from build123d import *

# Parameters (mm, degrees)
EXTRUDE002_DEPTH = 3
SKETCH001_W      = 60
SKETCH001_H      = 3
EXTRUDE001_DEPTH = 20
SKETCH_W         = 60
SKETCH_H         = 23
SKETCH_R         = 2.5
EXTRUDE_DEPTH    = 3


with BuildPart() as extrude002:
    # Face002 → Extrude002 (new body)
    with BuildSketch(Plane(origin=(30, 0, 17.604991), x_dir=(1, 0, 0), z_dir=(0, 1, 0))):
        with BuildLine():
            Line((-1, -5.395009), (1, -5.395009))
            Line((1, -5.395009), (1, 4.604991))
            ThreePointArc((1, 4.604991), (0, 5.604991), (-1, 4.604991))
            Line((-1, 4.604991), (-1, -5.395009))
        make_face()
    extrude(amount=EXTRUDE002_DEPTH)


with BuildPart() as cut:
    # Sketch001 (on Face7 of Extrude) → Extrude001 (new body)
    with BuildSketch(Plane.XY.offset(3)):
        with Locations((30, 1.5)):
            Rectangle(SKETCH001_W, SKETCH001_H)
    extrude(amount=EXTRUDE001_DEPTH)

    # Cut: cut Extrude002
    add(extrude002.part, mode=Mode.SUBTRACT)


with BuildPart() as fusion:
    # Sketch → Extrude (new body)
    with BuildSketch(Plane.XY):
        with Locations((30, 11.5)):
            Rectangle(SKETCH_W, SKETCH_H)
        with Locations((30, 13)):
            Circle(SKETCH_R, mode=Mode.SUBTRACT)
    extrude(amount=EXTRUDE_DEPTH)

    # Fusion: union Cut
    add(cut.part)


solid = fusion.part
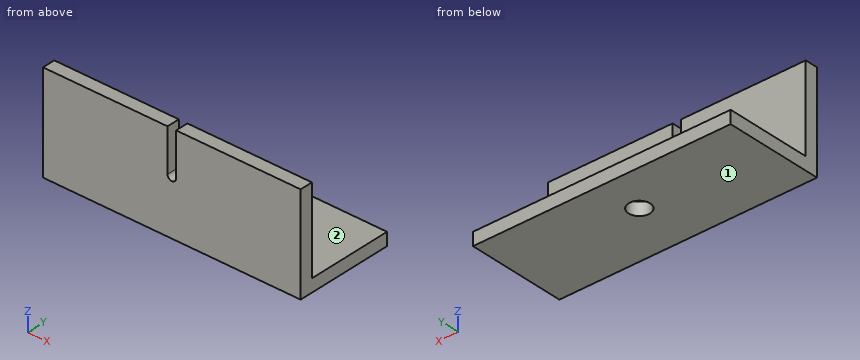
Source: CAD feature listing. Evaluate the final solid. Frame: model axes, mm. Face numbers are marked on the shaded views. A direction names the side the tool comes from. Give positions to 0.01 mm unless a question says otherwise; leave off trailing zeros. Order: outer loops, then holes, each group sorted by start corner. A loop starts at its lowest first (then second) coordinate and runs counter-clockwise, first axis right, second up. Notation, with made-up numbers: (81.5, 21.5) -> (93.5, 21.5) arc R29 cw to (93.5, 52.5) -> close; hole circle Ø9 at (65.5, 68). An arc over 180 degrees is marked (long way). Use a Markdown table: item, result.
1) Contact query for flat-ended pins moving along their axis: P1, Ø8, axis at x = 30, y = 13, coming from the +Z side; P2, Ø10, axis at x = 14.5, z = 11.5, coming from the +Y side; P3, Ø2.5, axis at y = 2, z = 20, coming from the -X side. Output: stop coordinate, or through.
Answer list:
| item | result |
|---|---|
| P1 | z = 3 |
| P2 | y = 3 |
| P3 | x = 0 |
2) Reachability of the marked faces 1 and 2 from +Z, -Z, +X, -X, +Y, -Y: full face, straight path, thin tool, end or side. Return the list, or none.
Answer list:
| item | result |
|---|---|
| face 1 | -Z, +X, -X, +Y, -Y |
| face 2 | +Z, +X, -X, +Y |
3) Section query B-B, the plane x = 30. Return the cut outline in (y, z), then the cut area to 3 significant figures.
Answer list:
| item | result |
|---|---|
| outline | (0, 0) -> (10.5, 0) -> (10.5, 3) -> (3, 3) -> (3, 12) -> (0, 12) -> close; (15.5, 0) -> (23, 0) -> (23, 3) -> (15.5, 3) -> close |
| area | 81.0 mm² |
4) Section query C-C, the plane y = 13. Return the cut outline in (x, z).
Answer list:
| item | result |
|---|---|
| outline | (0, 0) -> (27.5, 0) -> (27.5, 3) -> (0, 3) -> close; (32.5, 0) -> (60, 0) -> (60, 3) -> (32.5, 3) -> close |
5) Section query D-D, the plane x = 52.5. Return the cut outline in (y, z), then the cut area to 3 significant figures.
Answer list:
| item | result |
|---|---|
| outline | (0, 0) -> (23, 0) -> (23, 3) -> (3, 3) -> (3, 23) -> (0, 23) -> close |
| area | 129 mm² |
6) Ray query, line 1 along Y through (x, z) = (30, 0.75); line 2 along Z through (x, y) = (39, 13.75). Return the intervals inside material, ascending. Write a range as [from, to].
Answer list:
| item | result |
|---|---|
| line 1 | [0, 10.5], [15.5, 23] |
| line 2 | [0, 3] |
7) Section query A-A, the plane z = 14.75. Return the cut outline in (x, y), then the cut area to 3 significant figures.
Answer list:
| item | result |
|---|---|
| outline | (0, 0) -> (29, 0) -> (29, 3) -> (0, 3) -> close; (31, 0) -> (60, 0) -> (60, 3) -> (31, 3) -> close |
| area | 174 mm² |
